from build123d import *

# Parameters (mm, degrees)
SKETCH_W        = 72
SKETCH_H        = 41
PAD_DEPTH       = 2
POCKET_DEPTH    = 167.759861
SKETCH002_R     = 1.65
SKETCH002_W     = 3.5
SKETCH002_H     = 25.4
POCKET001_DEPTH = 2.001


with BuildPart() as part:
    # Sketch → Pad (new body)
    with BuildSketch(Plane.XY):
        Rectangle(SKETCH_W, SKETCH_H)
    extrude(amount=PAD_DEPTH)

    # Sketch001 (on Face6 of Pad) → Pocket (cut, through all)
    with BuildSketch(Plane.XY.offset(2)):
        with BuildLine():
            ThreePointArc((33.475, 16.5), (31.825, 18.15), (30.175, 16.5))
            Line((30.175, 16.5), (30.175, -16.5))
            ThreePointArc((30.175, -16.5), (31.825, -18.15), (33.475, -16.5))
            Line((33.475, 16.5), (33.475, -16.5))
        make_face()
    pocket = extrude(amount=-POCKET_DEPTH, mode=Mode.SUBTRACT)

    # Mirrored: Pocket across YZ
    add(pocket.mirror(Plane.YZ), mode=Mode.SUBTRACT)

    # Sketch002 (on Face5 of Mirrored) → Pocket001 (cut, through all)
    with BuildSketch(Plane.XY.offset(2)):
        with Locations((6, 7.75)):
            Circle(SKETCH002_R)
        with Locations((6, -7.75)):
            Circle(SKETCH002_R)
        with Locations((-6, 0)):
            Rectangle(SKETCH002_W, SKETCH002_H)
    extrude(amount=-POCKET001_DEPTH, mode=Mode.SUBTRACT)


solid = part.part
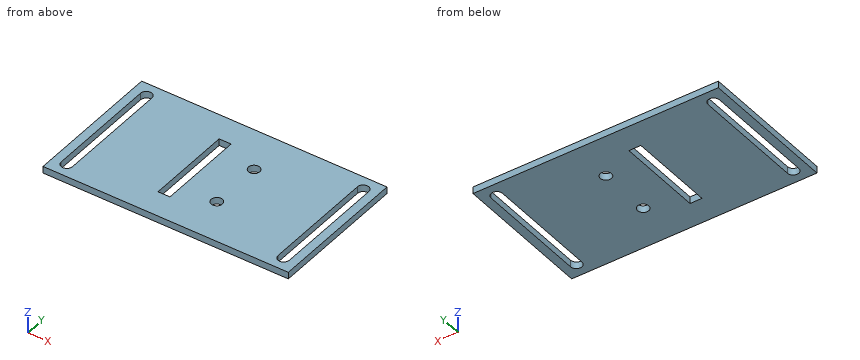
Verification items for the finished model (mm, model axes). Give positions to 0.01 mm unless a question says otherwise; leave off trailing zeros. Loops run counter-clockwise (first coordinate to the right, second up) from the corner with the lowest first, then second, coordinate; pieces in that order, holes last.
1. Cross-section at B-B on y = -11.5. Record the cut outline in (x, z) (3 decimals), and give its area (3 significant figures).
Derived:
outline: (-36, 0) - (-33.475, 0) - (-33.475, 2) - (-36, 2) - close; (-30.175, 0) - (-7.75, 0) - (-7.75, 2) - (-30.175, 2) - close; (-4.25, 0) - (30.175, 0) - (30.175, 2) - (-4.25, 2) - close; (33.475, 0) - (36, 0) - (36, 2) - (33.475, 2) - close
area: 124 mm2
2. Material ranges on probe 1 along Y at (x, z) = (6, 1.3); probe 2 along X at (y, z) = (-12, 0.15) (3 decimals); probe 3 along X at (y, z) = (-13, 0.45) (3 decimals), recorded low to high.
Derived:
probe 1: y = -20.5 to -9.4, -6.1 to 6.1, 9.4 to 20.5
probe 2: x = -36 to -33.475, -30.175 to -7.75, -4.25 to 30.175, 33.475 to 36
probe 3: x = -36 to -33.475, -30.175 to 30.175, 33.475 to 36
3. Cross-section at C-C on y = 7.75. Record the cut outline in (x, z) (3 decimals).
Derived:
outline: (-36, 0) - (-33.475, 0) - (-33.475, 2) - (-36, 2) - close; (-30.175, 0) - (-7.75, 0) - (-7.75, 2) - (-30.175, 2) - close; (-4.25, 0) - (4.35, 0) - (4.35, 2) - (-4.25, 2) - close; (7.65, 0) - (30.175, 0) - (30.175, 2) - (7.65, 2) - close; (33.475, 0) - (36, 0) - (36, 2) - (33.475, 2) - close
4. Cross-section at D-D on z = 0.35. Record the cut outline in (x, y) (3 decimals).
Derived:
outline: (-36, -20.5) - (36, -20.5) - (36, 20.5) - (-36, 20.5) - close; hole (-33.475, -16.5) arc R1.65 ccw to (-30.175, -16.5) - (-30.175, 16.5) arc R1.65 ccw to (-33.475, 16.5) - close; hole (-7.75, -12.7) - (-4.25, -12.7) - (-4.25, 12.7) - (-7.75, 12.7) - close; hole circle Ø3.3 at (6, -7.75); hole circle Ø3.3 at (6, 7.75); hole (30.175, -16.5) arc R1.65 ccw to (33.475, -16.5) - (33.475, 16.5) arc R1.65 ccw to (30.175, 16.5) - close
5. Go/stop test with a flat-tipped pin: P1, Ø2.5, axis at x = 6, y = -7.75, coming from the -Z side (3 decimals). Record where the tip stops, or that it passes through.
Derived:
P1: passes through
6. Cross-section at A-A on x = 6. Record the cut outline in (y, z), and give its area (3 significant figures).
Derived:
outline: (-20.5, 0) - (-9.4, 0) - (-9.4, 2) - (-20.5, 2) - close; (-6.1, 0) - (6.1, 0) - (6.1, 2) - (-6.1, 2) - close; (9.4, 0) - (20.5, 0) - (20.5, 2) - (9.4, 2) - close
area: 68.8 mm2
